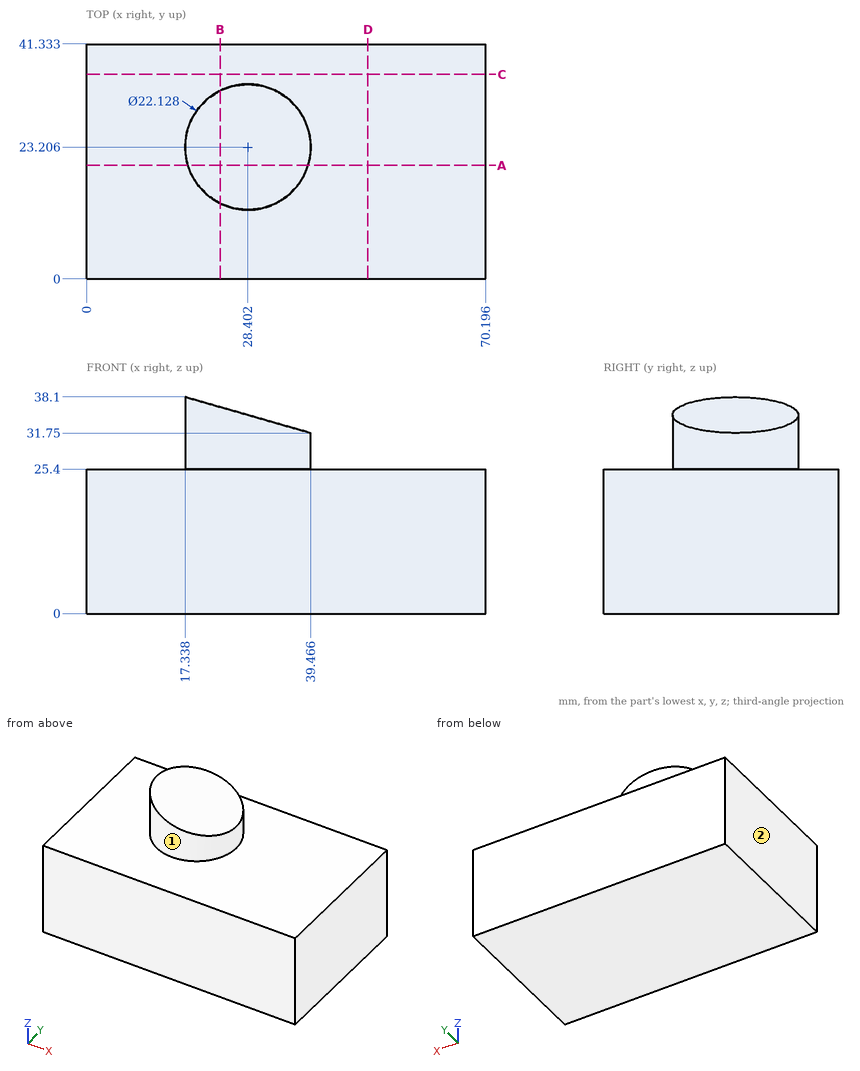
Design review of the part shown in the three views and the two pictorial views. Dimensions are in mm from the part's minimum x, y and z. A direction names the side the tool comes from. Coordinates: 2 decimals unless noted, no trailing zeros. Order: outer loops, then holes, each group sorted by start corner. A loop starts at its lowest first (then second) coordinate and runs counter-clockwise, first axis right, second up.
1) Take a section at B-B, the plane x = 23.5. Give the boundary of the cut face in (y, z) (1 decimal).
2) Take a section at A-A, the plane y = 20. Give the boundary of the cut face in (x, z), and give its area (3 significant figures).
3) Take a section at C-C, the plane y = 36. Give the boundary of the cut face in (x, z), and give its area (3 significant figures).
4) Take a section at D-D, the plane x = 49.5. Give the boundary of the cut face in (y, z).
5) Wall thickness on line 1 along Z through (x, y) = (67, 8.5); line 2 along Z through (x, y) = (26, 29) (1 decimal); line 3 along X through (y, z) = (19, 31) (1 decimal): over which ranges is each line inside the solid? List them lowest first.
6) For the marked faces 1 and 2, list the 3-axis set-ups (+Z, -Z, +X, -X, +Y, -Y) from which the entire face can be reached by the end or side of a thin tool; tool diameter is ignored.
7) Clearance check with a flat-ended pin moving along its axis: pin 1 (1.5 mm diameter, centred on x = 49, y = 35, fed in from +Z). State where the tip first meets the part, or that it passes through.
Returned:
1. outline: (0, 0) - (41.3, 0) - (41.3, 25.4) - (33.1, 25.4) - (33.1, 36.3) - (13.3, 36.3) - (13.3, 25.4) - (0, 25.4) - close
2. outline: (0, 0) - (70.2, 0) - (70.2, 25.4) - (38.99, 25.4) - (38.99, 31.89) - (17.81, 37.96) - (17.81, 25.4) - (0, 25.4) - close
2. area: 1,980 mm2
3. outline: (0, 0) - (70.2, 0) - (70.2, 25.4) - (0, 25.4) - close
3. area: 1,780 mm2
4. outline: (0, 0) - (41.33, 0) - (41.33, 25.4) - (0, 25.4) - close
5. line 1: z = 0 to 25.4
5. line 2: z = 0 to 35.6
5. line 3: x = 18.2 to 38.6
6. face 1: +Z
6. face 2: +Z, -Z, -X, +Y, -Y
7. pin 1: stops at z = 25.4
